from build123d import *

# Parameters (mm, degrees)
SKETCH_1_R               = 50.4
SKETCH_1_R_2             = 40.9
EXTRUDE_1_DEPTH          = 13
SKETCH_2_R               = 1
SKETCH_2_R_2             = 0.85
CUT_EXTRUDE_1_DEPTH      = 13
SKETCH_3_R               = 1.5
CUT_EXTRUDE_2_DEPTH      = 5
PATTERN_CIRCULAR_1_COUNT = 6


with BuildPart() as part:
    # 草图1 → 凸台-拉伸1 (new body)
    with BuildSketch(Plane(origin=(0, 0, 0), x_dir=(1, 0, 0), z_dir=(0, 1, 0))):
        with Locations(Location((0, 0, 0), (0, 0, 270))):
            Circle(SKETCH_1_R)
        with Locations(Location((0, 0, 0), (0, 0, 270))):
            Circle(SKETCH_1_R_2, mode=Mode.SUBTRACT)
    extrude(amount=-EXTRUDE_1_DEPTH)

    # 草图2 → 切除-拉伸1 (cut)
    with BuildSketch(Plane.XZ.offset(13)):
        with Locations((0, 50.4)):
            Circle(SKETCH_2_R)
        with Locations((50.4, 0)):
            Circle(SKETCH_2_R)
        with Locations((0, -50.4)):
            Circle(SKETCH_2_R)
        with Locations((-50.4, 0)):
            Circle(SKETCH_2_R)
        with Locations((-25.2, 43.647680351)):
            Circle(SKETCH_2_R_2)
        with Locations((25.2, 43.647680351)):
            Circle(SKETCH_2_R_2)
        with Locations((43.647680351, 25.2)):
            Circle(SKETCH_2_R_2)
        with Locations((43.647680351, -25.2)):
            Circle(SKETCH_2_R_2)
        with Locations((25.2, -43.647680351)):
            Circle(SKETCH_2_R_2)
        with Locations((-25.2, -43.647680351)):
            Circle(SKETCH_2_R_2)
        with Locations((-43.647680351, -25.2)):
            Circle(SKETCH_2_R_2)
        with Locations((-43.647680351, 25.2)):
            Circle(SKETCH_2_R_2)
    extrude(amount=-CUT_EXTRUDE_1_DEPTH, mode=Mode.SUBTRACT)

    # 草图3 → 切除-拉伸2 (cut)
    with BuildSketch(Plane(origin=(0, 0, 0), x_dir=(1, 0, 0), z_dir=(0, 1, 0))):
        with Locations(Location((-11.258628462, 42.017773444, 0), (0, 0, 270))):
            Circle(SKETCH_3_R)
    cut_extrude_2 = extrude(amount=-CUT_EXTRUDE_2_DEPTH, mode=Mode.SUBTRACT)

    # 阵列(圆周)1: 切除-拉伸2 ×6 about axis
    pattern_circular_1_axis = Axis((0, 0, 0), (0, 1, 0))
    for i in range(1, PATTERN_CIRCULAR_1_COUNT):
        add(cut_extrude_2.rotate(pattern_circular_1_axis, i * 360 / PATTERN_CIRCULAR_1_COUNT), mode=Mode.SUBTRACT)


solid = part.part
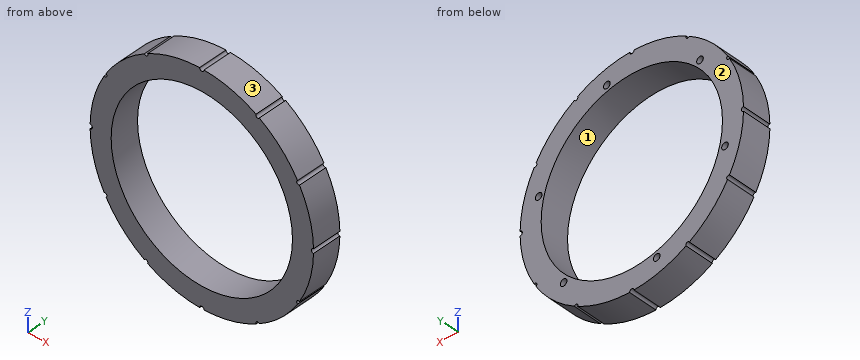
Check sheet for the modelled part. Datum: model origin and axes. Units: mm. Face numbers are marked on the shaded views. Round coordinates to 2 decimals unless told otherwise and drop trailing zeros. Loops run counter-clockwise (first coordinate to the right, second up) from the corner with the lowest first, then second, coordinate; pieces in that order, holes last.
1. Sectioned sample at A-A on z = -23. Record the boundary of the cut face in (x, y).
2. Sectioned sample at B-B on x = -6. Record the boundary of the cut face in (y, z), and give its area (3 significant figures).
3. Scan lines: probe 1 along X at (y, z) = (-1.75, 0); probe 2 along Z at (x, y) = (11.5, -1); probe 3 along Z at (x, y) = (-43, -1.5). Record each from-to range of solid material in increasing order.
4. Gauge pin test, flat ends, axial feed: pin 1 Ø5 at (y, z) = (-6.5, 39) entering from +X (3 decimals); pin 2 Ø1.5 at (y, z) = (-11, 2.5) entering from +X; pin 3 Ø1.8 at (x, z) = (-11.26, -42.02) entering from +Y. Record the tip position at first contact, or that the pin passes through.
5. Sectioned sample at C-C on y = -3.25. Give the number of separate pieces and of enclosed holes in the cut face, and give its area (3 significant figures).
6. Mould release check, pull along X, two halves, no side actions. Record for the marked faces 1, 2 and 3: released by +X, released by -X, zero draft, split by the parting line, or undercut.
Recorded:
1. outline: (-44.85, -13) - (-33.82, -13) - (-33.82, 0) - (-44.85, 0) - close; (33.82, -13) - (44.85, -13) - (44.85, 0) - (33.82, 0) - close
2. outline: (-13, -50.04) - (0, -50.04) - (0, -40.46) - (-13, -40.46) - close; (-13, 40.46) - (0, 40.46) - (0, 50.04) - (-13, 50.04) - close
2. area: 249 mm2
3. probe 1: x = -49.4 to -40.9, 40.9 to 49.4
3. probe 2: z = -49.07 to -39.25, 39.25 to 40.54, 43.5 to 49.07
3. probe 3: z = -26.29 to -25.75, -24.65 to -12.39, -10.12 to 24.65, 25.75 to 26.29
4. pin 1: stops at x = 34.755
4. pin 2: stops at x = 50.37
4. pin 3: stops at y = -5
5. separate pieces: 1
5. enclosed holes: 7
5. area: 2,670 mm2
6. face 1: undercut
6. face 2: zero draft
6. face 3: released by +X
